```python
from build123d import *

# Parameters (mm, degrees)
CROQUIS1_W              = 10
CROQUIS1_H              = 12.25
SALIENTE_EXTRUIR1_DEPTH = 6.5
CROQUIS2_W              = 7.4
CROQUIS2_H              = 6.875
CROQUIS2_R              = 1
SALIENTE_EXTRUIR2_DEPTH = 5.4
CROQUIS3_R              = 1
CROQUIS3_W              = 12.25
CROQUIS3_H              = 3.5
CORTAR_EXTRUIR1_DEPTH   = 35.4


with BuildPart() as part:
    # Croquis1 → Saliente-Extruir1 (new body)
    with BuildSketch(Plane(origin=(0, 0, 0), x_dir=(1, 0, 0), z_dir=(0, 1, 0))):
        Polygon((-15.606807411, 13.619327476), (-15.606807411, 6.744327476), (-9.43180722, 6.744327476), (-9.43180722, -5.505672524), (-15.606807411, -5.505672524), (-15.606807411, -12.380672524), (17.093193352, -12.380672524), (17.093193352, -5.505672524), (10.918193161, -5.505672524), (10.918193161, 6.744327476), (17.093193352, 6.744327476), (17.093193352, 13.619327476), align=None)
        with Locations((0.743192971, 0.619327476)):
            Rectangle(CROQUIS1_W, CROQUIS1_H, mode=Mode.SUBTRACT)
    extrude(amount=SALIENTE_EXTRUIR1_DEPTH)

    # Croquis2 → Saliente-Extruir2 (add)
    with BuildSketch(Plane(origin=(0, 6.5, 0), x_dir=(1, 0, 0), z_dir=(0, 1, 0))):
        with Locations((0.743192971, -8.943172524)):
            Rectangle(CROQUIS2_W, CROQUIS2_H)
        with Locations((0.743192971, -8.943172524)):
            Circle(CROQUIS2_R, mode=Mode.SUBTRACT)
        with Locations((0.743192971, 10.181827476)):
            Rectangle(CROQUIS2_W, CROQUIS2_H)
        with Locations((0.743192971, 10.181827476)):
            Circle(CROQUIS2_R, mode=Mode.SUBTRACT)
    extrude(amount=SALIENTE_EXTRUIR2_DEPTH)

    # Croquis3 → Cortar-Extruir1 (cut)
    with BuildSketch(Plane.ZY.offset(15.606807411)):
        with Locations((-10.181827476, 3.25)):
            Circle(CROQUIS3_R)
        with Locations((8.943172524, 3.25)):
            Circle(CROQUIS3_R)
        with Locations((-0.619327476, 4.75)):
            Rectangle(CROQUIS3_W, CROQUIS3_H)
    extrude(amount=-CORTAR_EXTRUIR1_DEPTH, mode=Mode.SUBTRACT)


solid = part.part
```
For this review, take the finished solid that the model builds, in its own axes (mm). A direction names the side the tool comes from. Round coordinates to 2 decimals unless told otherwise and drop trailing zeros. Write each loop counter-clockwise with the first axis right and the second up, starting at its lowest first coordinate (ties: lowest second). Pieces come first, ordered by that corner, then holes.
1) Take a section at D-D on y = 5.75. Give the boundary of the cut face in (x, z).
Answer below:
outline: (-15.61, -13.62) - (17.09, -13.62) - (17.09, -6.74) - (-15.61, -6.74) - close; (-15.61, 5.51) - (17.09, 5.51) - (17.09, 12.38) - (-15.61, 12.38) - close
2) Take a section at A-A on z = 1.25. Give the boundary of the cut face in (x, y).
Answer below:
outline: (-9.43, 0) - (-4.26, 0) - (-4.26, 3) - (-9.43, 3) - close; (5.74, 0) - (10.92, 0) - (10.92, 3) - (5.74, 3) - close
3) Take a section at B-B on y = 1.25. Give the boundary of the cut face in (x, z).
Answer below:
outline: (-15.61, -13.62) - (17.09, -13.62) - (17.09, -6.74) - (10.92, -6.74) - (10.92, 5.51) - (17.09, 5.51) - (17.09, 12.38) - (-15.61, 12.38) - (-15.61, 5.51) - (-9.43, 5.51) - (-9.43, -6.74) - (-15.61, -6.74) - close; hole (-4.26, -6.74) - (5.74, -6.74) - (5.74, 5.51) - (-4.26, 5.51) - close
4) For line 1 along Z through (x, y) = (-2.5, 7); line 2 along Z through (x, y) = (0, 11); line 3 along Z through (x, y) = (14.5, 4), list the stretches that pass through material, from the lowest coordinate up.
Answer below:
line 1: z = -13.62 to -6.74, 5.51 to 12.38
line 2: z = -13.62 to -10.85, -9.51 to -6.74, 5.51 to 8.27, 9.61 to 12.38
line 3: z = -13.62 to -10.84, -9.52 to -6.74, 5.51 to 8.28, 9.6 to 12.38
5) Insertion check: pin 1 Ø4 at (x, z) = (-8, -0.5) entering from +Y; pin 2 Ø1 at (x, z) = (1, 9) entering from +Y; pin 3 Ø1.5 at (y, z) = (2, 1) entering from -X. Each pin has a flat end and moves straight along its axis. Give the tip position at first contact, or say it passes through.
Answer below:
pin 1: stops at y = 3
pin 2: stops at y = 6.5
pin 3: stops at x = -9.43
6) Take a section at C-C on x = -1. Give the boundary of the cut face in (y, z).
Answer below:
outline: (0, -13.62) - (11.9, -13.62) - (11.9, -6.74) - (0, -6.74) - close; (0, 5.51) - (11.9, 5.51) - (11.9, 12.38) - (0, 12.38) - close; hole circle Ø2 at (3.25, -10.18); hole circle Ø2 at (3.25, 8.94)
7) Machinability: for faces 1 (the face through (1, 5, -6.744)), 2 (the face through (-9, 6.5, 9)), 3 (the face through (11, 6.5, 9)), 4 (the face through (-4.257, 1, -1)), which of the approach directions +Z, -Z, +X, -X, +Y, -Y give a long, thin tool a straight path to every point of the face, cutting with its end or side? Answer none if there is none.
Answer below:
face 1: +Y
face 2: +Z, -Z, -X, +Y
face 3: +Z, -Z, +X, +Y
face 4: +Y, -Y
8) Mouldability with a two-part tool opening along Z and no side actions: class faces 5 (the face through (0.514, 4.093, 9.481)), 6 (the face through (1, 5, 12.381)), 7 (the face through (-15.607, 2, -11)) as +Z half, -Z half, draft (parallel to the pull), parting line (faces both ways), or undercut.
Answer below:
face 5: undercut
face 6: +Z half
face 7: draft
